Can you work these out from the model? Positions are in its coordinate system, mm. A direction names the side the tool comes from. Coordinates: 2 decimals unless noted, no trailing zeros. Order: outer loops, then holes, each group sorted by start corner. A loop starts at its lowest first (then second) coordinate and runs counter-clockwise, first axis right, second up. Notation, with made-up numbers: (33.25, -39) -> (68.25, -39) arc R15 ccw to (68.25, -35) -> close; hole circle Ø7 at (41, 13). An arc over 180 degrees is marked (long way). Answer as a JSON object with one key per item and string values. Group by question number.
(1) Which directions (+Z, -Z, +X, -X, +Y, -Y) give clear straight access to the entire face, cutting with the end or side of a thin tool? Please do faces 5 (the cylindrical face through (2169.77, 314.42, 737.93)), 6 (the cylindrical face through (1785.461, 1271.885, 1028.61)), 7 (the flat face through (2117, 544, 307.139)).
(2) I want a section at A-A, the plane z = 580.5. List the corners of the cut face in (x, y) for me.
(3) If we mould it in two halves opening along Z, with no side actions, what happens to faces 1 (the flat face through (2134, -520.7, 528)), 2 (the flat face through (2117, 549, 759.661)), 3 (the cylindrical face through (2145.59, -482.51, 36.215)), 4 (the cylindrical face through (2057.5, 777.78, 328.87))? For each: pulls with the +Z half, pulls with the -Z half, needs draft (parallel to the pull), parting line crosses it, or undercut.
(4) I want a section at B-B, the plane z = 219.5. List the corners of the cut face in (x, y) for me.
(5) I want a section at C-C, the plane x = 1845. List the corners of the cut face in (y, z) for me.
(6) I need wall thicknesses on line 1 (X direction, y = -364.5, z = 338.5); line 2 (X direction, y = 365, z = 227.5); line 3 (Z direction, x = 1845, y = 1204.5). Which ranges of each line are inside material? Lowest first, please.
(7) I want a section at D-D, the plane y = -330. List the corners of the cut face in (x, z) for me.
(8) For pin 1 (5 mm diameter, centred on y = 712.5, z = 260, fed in from +X); pin 2 (8 mm diameter, centred on y = 956, z = 114, fed in from +X); pin 3 (3 mm diameter, centred on x = 1871, z = 227, fed in from -Y), each with a flat end and sliding along its axis, tell me the tip position at first contact or that it passes through.
from build123d import *

# Parameters (mm, degrees)
BOSS_EXTRUDE2_DEPTH     = 1066.8
CUT_EXTRUDE1_DEPTH      = 2806.00308884
CUT_EXTRUDE1_DEPTH_BACK = 2806.00308884
FILLET1_R               = 127


with BuildPart() as part:
    # Sketch1 → Boss-Extrude2 (new body)
    with BuildSketch(Plane.XY):
        with BuildLine():
            Line((1708.013552171, 1308.1), (1818.71626935, 1308.1))
            ThreePointArc((1818.71626935, 1308.1), (2198.04838822, 432.940829033), (2178.927715276, -520.7))
            Line((2178.927715276, -520.7), (2087.416444891, -520.7))
            ThreePointArc((2087.416444891, -520.7), (2106.525474721, 437.019826496), (1708.013552171, 1308.1))
        make_face()
    extrude(amount=BOSS_EXTRUDE2_DEPTH)

    # Sketch2 → Cut-Extrude1 (cut, two sides: drawn at the far end of the back side and taken through both)
    with BuildSketch(Plane(origin=(0, 0, 0), x_dir=(0, 0, -1), z_dir=(1, 0, 0)).offset(-CUT_EXTRUDE1_DEPTH_BACK)):
        with BuildLine():
            Line((-683.460599828, 291.508156212), (-383.339400172, 291.508156212))
            ThreePointArc((-383.339400172, 291.508156212), (-329.457863446, 313.826619486), (-307.139400172, 367.708156212))
            Line((-307.139400172, 367.708156212), (-307.139400172, 724.491843788))
            ThreePointArc((-307.139400172, 724.491843788), (-329.457863446, 778.373380514), (-383.339400172, 800.691843788))
            Line((-383.339400172, 800.691843788), (-683.460599828, 800.691843788))
            ThreePointArc((-683.460599828, 800.691843788), (-737.342136554, 778.373380514), (-759.660599828, 724.491843788))
            Line((-759.660599828, 724.491843788), (-759.660599828, 367.708156212))
            ThreePointArc((-759.660599828, 367.708156212), (-737.342136554, 313.826619486), (-683.460599828, 291.508156212))
        make_face()
    extrude(amount=CUT_EXTRUDE1_DEPTH + CUT_EXTRUDE1_DEPTH_BACK, mode=Mode.SUBTRACT)

    # Fillet1
    fillet1_edges = [part.edges().sort_by_distance(p)[0] for p in [
        (2133.172080084, -520.7, 1066.8),
        (2133.172080084, -520.7, 0),
        (1763.364910761, 1308.1, 0),
        (1763.364910761, 1308.1, 1066.8),
    ]]
    fillet(fillet1_edges, radius=FILLET1_R)


solid = part.part
Computed values:
{
 "1": {"face 5": "+X, -X, +Y", "face 6": "+Z, +X, -X, +Y", "face 7": "+X, -X"},
 "2": {"outline": "(1708.01, 1308.1) arc R2151.38 cw to (1996.83, 800.69) -> (2092.31, 800.69) arc R2240.28 ccw to (1818.72, 1308.1) -> close; (2087.42, -520.7) -> (2178.93, -520.7) arc R2240.28 ccw to (2221.23, 291.51) -> (2131.54, 291.51) arc R2151.38 cw to start"},
 "3": {"face 1": "needs draft", "face 2": "undercut", "face 3": "pulls with the -Z half", "face 4": "undercut"},
 "4": {"outline": "(1708.01, 1308.1) arc R2151.38 cw to (2087.42, -520.7) -> (2178.93, -520.7) arc R2240.28 ccw to (1818.72, 1308.1) -> close"},
 "5": {"outline": "(1106.53, 0) -> (1181.1, 0) arc R127 ccw to (1270.76, 37.05) -> (1270.76, 1029.75) arc R127 ccw to (1181.1, 1066.8) -> (1106.53, 1066.8) -> close"},
 "6": {"line 1": "x = 2120.28 to 2210.43", "line 2": "x = 2120.19 to 2210.35", "line 3": "z = 2.17 to 1064.63"},
 "7": {"outline": "(2125.92, 0) -> (2215.84, 0) -> (2215.84, 1066.8) -> (2125.92, 1066.8) -> close"},
 "8": {"pin 1": "stops at x = 2124.8", "pin 2": "stops at x = 2027.94", "pin 3": "stops at y = 1059.33"}
}
